```python
from build123d import *

# Parameters (mm, degrees)
F0_R      = 99.06
F1_DEPTH  = 309.88
F1_FACE_R = 99.06
F2_DEPTH  = 1242.06
F3_SIZE   = 5.08
F4_SIZE   = 5.08


with BuildPart() as f1:
    # F0 (on Top) → F1 (new body)
    with BuildSketch(Plane.XY):
        Circle(F0_R)
    extrude(amount=F1_DEPTH)

    # F1_face (on face) → F2 (join)
    with BuildSketch(Plane(origin=(0, 0, 0), x_dir=(1, 0, 0), z_dir=(0, 0, -1))):
        Circle(F1_FACE_R)
    extrude(amount=F2_DEPTH)

    # F3
    f3_edges = [f1.edges().sort_by_distance(p)[0] for p in [
        (-99.06, 0, -1242.06),
    ]]
    chamfer(f3_edges, length=F3_SIZE)

    # F4
    f4_edges = [f1.edges().sort_by_distance(p)[0] for p in [
        (-99.06, 0, 309.88),
    ]]
    chamfer(f4_edges, length=F4_SIZE)


solid = f1.part
```
Read the model definition and answer for the solid it produces. Units are mm, in the model's axes. Round coordinates to 2 decimals unless told otherwise and drop trailing zeros. Write each loop counter-clockwise with the first axis right and the second up, starting at its lowest first coordinate (ties: lowest second). Pieces come first, ordered by that corner, then holes. Notation, with made-up numbers: (-14, -37) - (-5, -37) arc R7 cw to (-5, -25) - close; hole circle Ø3 at (20, 80.5). An arc over 180 degrees is marked (long way). Use CSV: the item, a comma, the result in double quotes.
Q1. Straight lines are drawn through the part: line 1 along Y through (x, z) = (-2.5, 64.5); line 2 along X through (y, z) = (3, 64.5); line 3 along X through (y, z) = (31.5, -805.5). For each, find the intervals that lie inside material, in ascending order.
Values:
line 1,"y = -99.03 to 99.03"
line 2,"x = -99.01 to 99.01"
line 3,"x = -93.92 to 93.92"
Q2. Each of these flat-tipped pins is pushed along its axis until it touches: pin 1 Ø12 at (x, z) = (78.5, -1085) entering from -Y; pin 2 Ø1 at (x, z) = (-2.5, 19) entering from -Y; pin 3 Ø12 at (y, z) = (71.5, -708.5) entering from +X. Where does it stop, or does it pass through?
Values:
pin 1,"stops at y = -67.5"
pin 2,"stops at y = -99.04"
pin 3,"stops at x = 74.31"
Q3. Find section A-A, the plane z = -64. Write down the section's boundary in (x, y), then the cut area to 3 significant figures.
Values:
outline,"circle Ø198.12 at (0, 0)"
area,"30,800 mm²"
